Input: part model. Units: mm. Frame: model coordinates. Face numbers are marked on the shaded views. A direction names the side the tool comes from. Give positions to 0.01 mm unless a question says otherwise; leave off trailing zeros. Order: outer loops, then holes, each group sorted by start corner. A loop starts at its lowest first (then second) coordinate and runs counter-clockwise, first axis right, second up. Notation, with made-up numbers: (6.5, 80) - (22.5, 80) arc R23 cw to (22.5, 112) - close; hole circle Ø9 at (76.5, 11). An arc over 180 degrees is marked (long way). Answer in a Markdown table with one row per item. Add a question column.
from build123d import *

# Parameters (mm, degrees)
SKETCH2_R           = 16.5
SKETCH2_R_2         = 12.5
SKETCH2_R_3         = 7.25
BOSS_EXTRUDE1_DEPTH = 4
BOSS_EXTRUDE3_START = -67
SKETCH2_4_R         = 16.5
SKETCH2_4_R_2       = 12.5
BOSS_EXTRUDE3_DEPTH = 67
SKETCH3_W           = 45
SKETCH3_H           = 45
BOSS_EXTRUDE4_DEPTH = 4
CHAMFER1_SIZE       = 10


with BuildPart() as part:
    # Sketch2 → Boss-Extrude1 (new body)
    # profile 1 of 2: a face of its own
    with BuildSketch(Plane(origin=(0, 0, 0), x_dir=(1, 0, 0), z_dir=(0, 1, 0))):
        with Locations(Location((0, 0, 0), (0, 0, 270))):
            Circle(SKETCH2_R)
        Circle(SKETCH2_R_2, mode=Mode.SUBTRACT)
    # profile 2 of 2: a face of its own
    with BuildSketch(Plane(origin=(0, 0, 0), x_dir=(1, 0, 0), z_dir=(0, 1, 0))):
        Circle(SKETCH2_R_2)
        with Locations(Location((0, 0, 0), (0, 0, 270))):
            Circle(SKETCH2_R_3, mode=Mode.SUBTRACT)
    extrude(amount=BOSS_EXTRUDE1_DEPTH)

    # Sketch2<4> → Boss-Extrude3 (add)
    with BuildSketch(Plane(origin=(0, 0, 0), x_dir=(1, 0, 0), z_dir=(0, 1, 0)).offset(BOSS_EXTRUDE3_START)):
        with Locations(Location((0, 0, 0), (0, 0, 270))):
            Circle(SKETCH2_4_R)
        with Locations(Location((0, 0, 0), (0, 0, 270))):
            Circle(SKETCH2_4_R_2, mode=Mode.SUBTRACT)
    extrude(amount=BOSS_EXTRUDE3_DEPTH)

    # Sketch3 → Boss-Extrude4 (add)
    with BuildSketch(Plane(origin=(0, -67, 0), x_dir=(-1, 0, 0), z_dir=(0, -1, 0))):
        Rectangle(SKETCH3_W, SKETCH3_H)
    extrude(amount=BOSS_EXTRUDE4_DEPTH)

    # Chamfer1
    # the kernel refuses this chamfer: 10 mm, written as the material it adds along each edge
    with BuildSketch(Plane(origin=(0, -67, 0), x_dir=(0, 0, 1), z_dir=(-1, 0, 0))) as chamfer1_piece_1_section:
        Polygon((16.5 + CHAMFER1_SIZE, 0), (16.5, CHAMFER1_SIZE), (16.5, 0), align=None)
    chamfer1_piece_1 = revolve(axis=Axis((0, -67, 0), (0, 1, 0)), mode=Mode.PRIVATE)
    chamfer1_piece_1 = split(chamfer1_piece_1, bisect_by=Plane(origin=(0, -62.130236746, -22.5), z_dir=(0, 0, 1)), keep=Keep.TOP, mode=Mode.PRIVATE)
    chamfer1_piece_1 = split(chamfer1_piece_1, bisect_by=Plane(origin=(22.5, -62.130236746, -21.369763254), z_dir=(-1, 0, 0)), keep=Keep.TOP, mode=Mode.PRIVATE)
    chamfer1_piece_1 = split(chamfer1_piece_1, bisect_by=Plane(origin=(-22.5, -62.130236746, -21.369763254), z_dir=(1, 0, 0)), keep=Keep.TOP, mode=Mode.PRIVATE)
    chamfer1_piece_1 = split(chamfer1_piece_1, bisect_by=Plane(origin=(0, -62.130236746, 22.5), z_dir=(0, 0, -1)), keep=Keep.TOP, mode=Mode.PRIVATE)
    add(chamfer1_piece_1)


solid = part.part
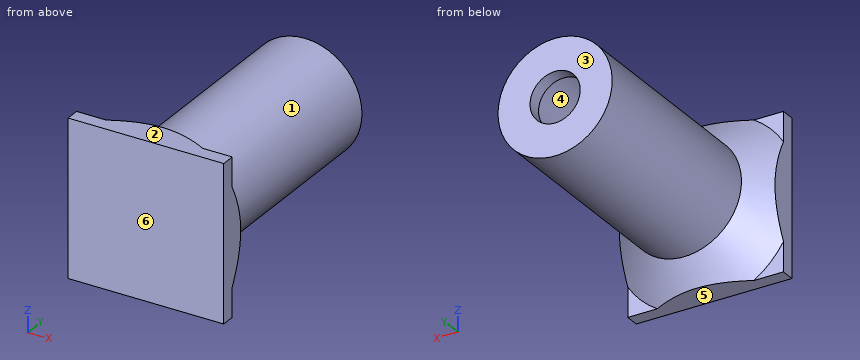
Q1. Section B-B, the plane x = 0. Return loops of the section in (y, z).
Q2. Section A-A, the plane z = 0. Return loops of the section in (x, y).
Q3. Contact query for flat-ended pins moving along their axis: P1, Ø8.5, axis at x = 0, z = 0, coming from the +Y side; P2, Ø9.5, axis at x = 16.5, z = 16.5, coming from the +Y side; P3, Ø8, axis at x = 0.5, y = -23.5, coming from the -Z side. Output: stop coordinate, or through.
Q4. Pull-direction query (Y, two-part tool) for the marked faces 3, 4, 5 and 6; classes: +Y half, -Y half, draft (parallel to the pull), parting line (faces both ways), or undercut.
Q5. Access query for the marked faces 1 and 2. Directions: +Z, -Z, +X, -X, +Y, -Y. A direction counts if a zero-diameter tool reaches every point of the face in a straight line with its end or side. Return the directions, or none.
Q6. Line query: probe 1 along Y at (x, z) = (-6, 9); probe 2 along X at (y, z) = (2, 0); probe 3 along X at (y, z) = (-26.5, 1). Output: solid intervals per line, ascending.
Q7. Section C-C, the plane y = -26.5. Return loops of the section in (x, z).
Computed:
| question | item | result |
|---|---|---|
| 1 | outline | (-71, -22.5) - (-63, -22.5) - (-57, -16.5) - (4, -16.5) - (4, -7.25) - (0, -7.25) - (0, -12.5) - (-67, -12.5) - (-67, 12.5) - (0, 12.5) - (0, 7.25) - (4, 7.25) - (4, 16.5) - (-57, 16.5) - (-63, 22.5) - (-71, 22.5) - close |
| 2 | outline | (-22.5, -71) - (22.5, -71) - (22.5, -63) - (16.5, -57) - (16.5, 4) - (7.25, 4) - (7.25, 0) - (12.5, 0) - (12.5, -67) - (-12.5, -67) - (-12.5, 0) - (-7.25, 0) - (-7.25, 4) - (-16.5, 4) - (-16.5, -57) - (-22.5, -63) - close |
| 3 | P1 | stops at y = -67 |
| 3 | P2 | stops at y = -59.08 |
| 3 | P3 | stops at z = -16.5 |
| 4 | face 3 | +Y half |
| 4 | face 4 | undercut |
| 4 | face 5 | draft |
| 4 | face 6 | -Y half |
| 5 | face 1 | +Y |
| 5 | face 2 | +Z, +X, -X, +Y, -Y |
| 6 | probe 1 | y = -71 to -67, 0 to 4 |
| 6 | probe 2 | x = -16.5 to -7.25, 7.25 to 16.5 |
| 6 | probe 3 | x = -16.47 to -12.46, 12.46 to 16.47 |
| 7 | outline | circle Ø33 at (0, 0); hole circle Ø25 at (0, 0) |
